The listing builds one solid part. Answer for the finished solid, in the listing's coordinates (mm). Face numbers are marked on the shaded views. A direction names the side the tool comes from. Give positions to 0.01 mm unless a question says otherwise; leave off trailing zeros. Write each loop counter-clockwise with the first axis right and the second up, starting at its lowest first coordinate (ties: lowest second). Pieces come first, ordered by that corner, then holes. Notation, with made-up numbers: (43, -26) -> (52, -26) arc R19 ccw to (52, -15) -> close; hole circle Ø6 at (33.25, -34.75). An arc over 180 degrees is marked (long way). Put each result on its own line as item: value. Start each with the question number.
1) For a pull along X with two mould halves and no side action, classify the marked faces 3 and 4 as released by +X, released by -X, zero draft, split by the parting line, or undercut.
2) A cutting plane is placed at D-D (z = -86.5). Write down the section's boundary in (x, y), then the cut area to 3 significant figures.
3) A cutting plane is placed at B-B (y = 7.5). Write down the section's boundary in (x, z), then the cut area to 3 significant figures.
4) Find the intervals of material crossed by line 1 along Y through (x, z) = (0, 55.5); line 2 along Y through (x, z) = (0.5, 15); line 3 along Z through (x, y) = (13, 10), in increasing order. Write a range as from..to.
5) Flat-ended cylindrical pins translate along their axes: pin 1 Ø1.5 at (x, z) = (4, -17.5) entering from -Y; pin 2 Ø6 at (x, z) = (5, -63) entering from +Y; pin 3 Ø3 at (y, z) = (2.5, 59.5) entering from -X; pin 4 Ø8 at (x, y) = (3, 7) entering from +Z. Find the tip coordinate at first contact, or state that the pin passes through.
6) For the marked faces 1 and 2, determine the directions among +Z, -Z, +X, -X, +Y, -Y from which every point of the face is accessible in a straight line to the end or side of a thin tool.
7) A cutting plane is placed at A-A (x = 0). Write down the section's boundary in (y, z), then the cut area to 3 significant figures.
8) A cutting plane is placed at C-C (z = -33.5). Write down the section's boundary in (x, y).
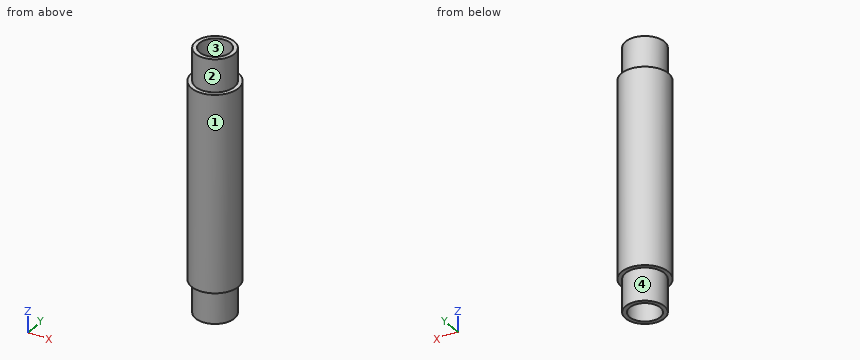
from build123d import *

# Parameters (mm, degrees)
SKETCH1_R           = 15.08125
SKETCH1_R_2         = 11.90625
BOSS_EXTRUDE1_DEPTH = 101.6
SKETCH2_R           = 18.25625
SKETCH2_R_2         = 11.90625
BOSS_EXTRUDE2_DEPTH = 76.2


with BuildPart() as part:
    # Sketch1 → Boss-Extrude1 (new, symmetric)
    with BuildSketch(Plane.XY):
        Circle(SKETCH1_R)
        Circle(SKETCH1_R_2, mode=Mode.SUBTRACT)
    extrude(amount=BOSS_EXTRUDE1_DEPTH, both=True)

    # Sketch2 → Boss-Extrude2 (add, symmetric)
    with BuildSketch(Plane.XY):
        with Locations(Location((0, 0, 0), (0, 0, 180))):
            Circle(SKETCH2_R)
        Circle(SKETCH2_R_2, mode=Mode.SUBTRACT)
    extrude(amount=BOSS_EXTRUDE2_DEPTH, both=True)


solid = part.part
Reply:
1. face 3: undercut
1. face 4: split by the parting line
2. outline: circle Ø30.16 at (0, 0); hole circle Ø23.81 at (0, 0)
2. area: 269 mm2
3. outline: (-16.64, -76.2) -> (-13.08, -76.2) -> (-13.08, -101.6) -> (-9.25, -101.6) -> (-9.25, 101.6) -> (-13.08, 101.6) -> (-13.08, 76.2) -> (-16.64, 76.2) -> close; (9.25, -101.6) -> (13.08, -101.6) -> (13.08, -76.2) -> (16.64, -76.2) -> (16.64, 76.2) -> (13.08, 76.2) -> (13.08, 101.6) -> (9.25, 101.6) -> close
3. area: 2,640 mm2
4. line 1: y = -18.26..-11.91, 11.91..18.26
4. line 2: y = -18.25..-11.9, 11.9..18.25
4. line 3: z = -76.2..76.2
5. pin 1: stops at y = -17.96
5. pin 2: stops at y = 18.15
5. pin 3: stops at x = -18.23
5. pin 4: passes through
6. face 1: +Z, -Z
6. face 2: +Z
7. outline: (-18.26, -76.2) -> (-15.08, -76.2) -> (-15.08, -101.6) -> (-11.91, -101.6) -> (-11.91, 101.6) -> (-15.08, 101.6) -> (-15.08, 76.2) -> (-18.26, 76.2) -> close; (11.91, -101.6) -> (15.08, -101.6) -> (15.08, -76.2) -> (18.26, -76.2) -> (18.26, 76.2) -> (15.08, 76.2) -> (15.08, 101.6) -> (11.91, 101.6) -> close
7. area: 2,260 mm2
8. outline: circle Ø36.51 at (0, 0); hole circle Ø23.81 at (0, 0)
